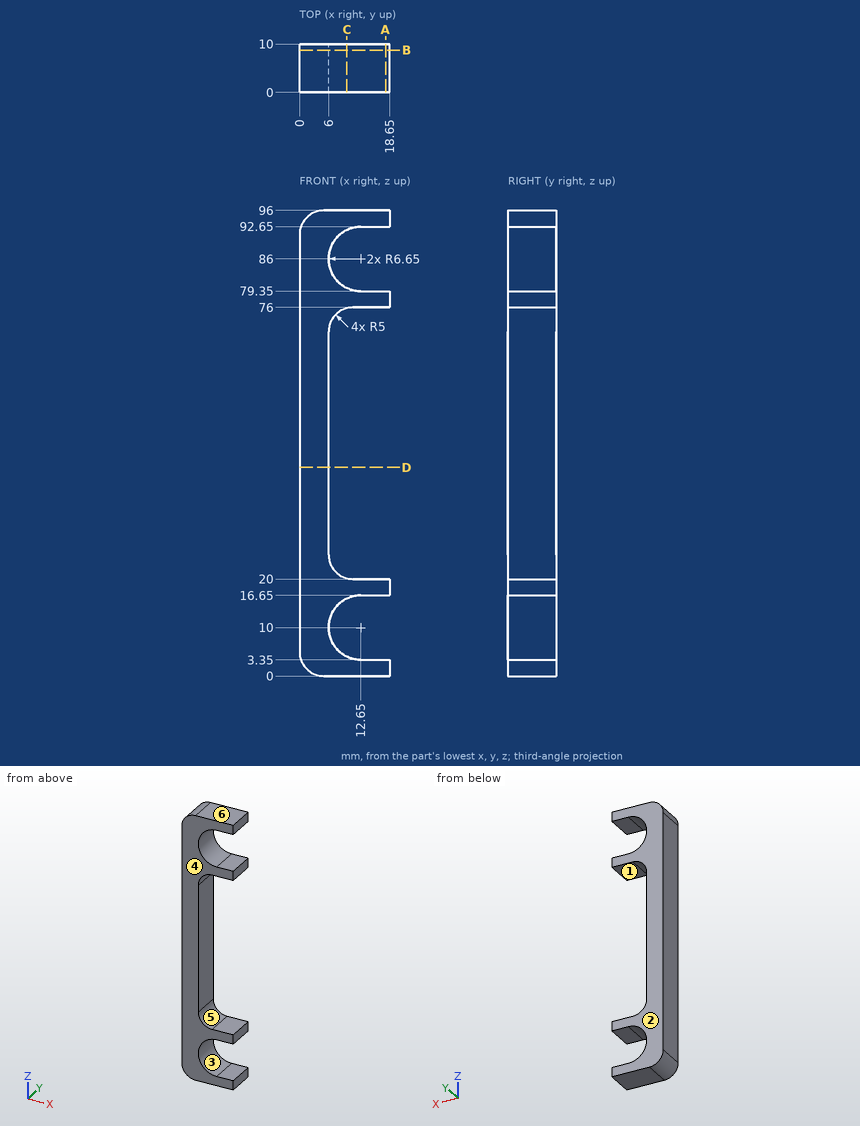
Input: dimensioned drawing with shaded views. Units: mm. Origin: part minimum x, y, z. A direction names the side the tool comes from. Round coordinates to 2 decimals unless told otherwise and drop trailing zeros. Order: outer loops, then holes, each group sorted by start corner. A loop starts at its lowest first (then second) coordinate and runs counter-clockwise, first axis right, second up. Notation, with made-up numbers: (32, 86.25) - (90, 86.25) arc R16 ccw to (90, 103.25) - close; hole circle Ø3 at (25, 39). An arc over 180 degrees is marked (long way). Use CSV: the item, a comma, the result in double quotes. Start each with the question number.
Q1. Mould query, pull axis Z, two halves, no side actions, for the marked faces 3, 4, 5 and 6. Classes: +Z half, -Z half, draft (parallel to the pull), parting line (faces both ways), or undercut.
Q2. Section query B-B (y = 8.75). Return loops of the section in (x, z).
Q3. First-contact query: pin 1 (8 mm diameter, centred on x = 12.5, z = 56.5, fed in from +Y); pin 2 (3 mm diameter, centred on y = 6, z = 53.5, fed in from +X). Flat tips, straight axial feed; report the tip coordinate or a pass-through.
Q4. Section query C-C (x = 9.75). Return loops of the section in (y, z), and give its area (3 significant figures).
Q5. Section query D-D (z = 43). Return loops of the section in (x, y).
Q6. Section query A-A (x = 17.75). Return loops of the section in (y, z).
Q7. Material intervals for line 1 along Z through (x, y) = (13.25, 6.75); line 2 along Z through (x, y) = (9.5, 3.5); line 3 along X through (y, z) = (4, 70), sorted ascending. Write a range as from..to.
Q8. Access query for the marked faces 1 and 2. Directions: +Z, -Z, +X, -X, +Y, -Y. A direction counts if a zero-diameter tool reaches every point of the face in a straight line with its end or side. Return the directions, or none.
Result set:
1,face 3,"undercut"
1,face 4,"draft"
1,face 5,"undercut"
1,face 6,"+Z half"
2,outline,"(0, 5) arc R5 ccw to (5, 0) - (18.65, 0) - (18.65, 3.35) - (12.65, 3.35) arc R6.65 cw to (12.65, 16.65) - (18.65, 16.65) - (18.65, 20) - (11, 20) arc R5 cw to (6, 25) - (6, 71) arc R5 cw to (11, 76) - (18.65, 76) - (18.65, 79.35) - (12.65, 79.35) arc R6.65 cw to (12.65, 92.65) - (18.65, 92.65) - (18.65, 96) - (5, 96) arc R5 ccw to (0, 91) - close"
3,pin 1,"passes through"
3,pin 2,"stops at x = 6"
4,outline,"(0, 0) - (10, 0) - (10, 4.02) - (0, 4.02) - close; (0, 15.98) - (10, 15.98) - (10, 20.16) - (0, 20.16) - close; (0, 75.84) - (10, 75.84) - (10, 80.02) - (0, 80.02) - close; (0, 91.98) - (10, 91.98) - (10, 96) - (0, 96) - close"
4,area,"164 mm2"
5,outline,"(0, 0) - (6, 0) - (6, 10) - (0, 10) - close"
6,outline,"(0, 0) - (10, 0) - (10, 3.35) - (0, 3.35) - close; (0, 16.65) - (10, 16.65) - (10, 20) - (0, 20) - close; (0, 76) - (10, 76) - (10, 79.35) - (0, 79.35) - close; (0, 92.65) - (10, 92.65) - (10, 96) - (0, 96) - close"
7,line 1,"z = 0..3.35, 16.65..20, 76..79.35, 92.65..96"
7,line 2,"z = 0..4.14, 15.86..20.23, 75.77..80.14, 91.86..96"
7,line 3,"x = 0..6"
8,face 1,"+X, +Y, -Y"
8,face 2,"+Z, -Z, +X, -X, +Y"
